The listing builds one solid part. Answer for the finished solid, in the listing's coordinates (mm). A direction names the side the tool comes from. Coordinates: 2 decimals unless noted, no trailing zeros. Order: outer loops, then holes, each group sorted by start corner. A loop starts at its lowest first (then second) coordinate and runs counter-clockwise, first axis right, second up. Notation, with made-up numbers: (-39, 44) -> (11, 44) arc R22 ccw to (11, 80) -> close; hole circle Ø4 at (68, 18.5). An arc over 180 degrees is marked (long way). Put each result on its own line as item: value. Start each with the question number.
```python
from build123d import *

# Parameters (mm, degrees)
CUT_EXTRUDE1_START = -2.681222
CUT_EXTRUDE1_DEPTH = 2.681222
CIRPATTERN3_COUNT  = 10
CUT_EXTRUDE2_REACH = 4.151
SKETCH5_R          = 2.323


with BuildPart() as part:
    # Sketch2 → Revolve2 (revolve)
    with BuildSketch(Plane(origin=(0, 0, 0), x_dir=(0, 0, -1), z_dir=(1, 0, 0))):
        Polygon((0, 0), (-7.8982, 0), (-9.91802604, 2.01982604), (-8.078303901, 3.859548179), (-6.369990486, 2.151234764), (0, 2.151234764), align=None)
    revolve(axis=Axis((0, 2.151234764, 0), (0, -1, 0)))

    # Sketch4 → Cut-Extrude1 (cut)
    with BuildSketch(Plane(origin=(-3.9491, -3.9491, 0), x_dir=(0, 0, 1), z_dir=(-0.707106781, -0.707106781, 0)).offset(CUT_EXTRUDE1_START)):
        with BuildLine():
            Line((-1.1615, 6.535539097), (1.1615, 6.535539097))
            ThreePointArc((1.1615, 6.535539097), (1.823938006, 9.981104914), (3.7168, 12.935393557))
            Line((3.7168, 12.935393557), (-3.7168, 12.935393557))
            ThreePointArc((-3.7168, 12.935393557), (-1.823938006, 9.981104914), (-1.1615, 6.535539097))
        make_face()
    cut_extrude1 = extrude(amount=CUT_EXTRUDE1_DEPTH, mode=Mode.SUBTRACT)

    # CirPattern3: Cut-Extrude1 ×10 about axis
    cirpattern3_axis = Axis((0, 0, 0), (0, 1, 0))
    for i in range(1, CIRPATTERN3_COUNT):
        add(cut_extrude1.rotate(cirpattern3_axis, i * 360 / CIRPATTERN3_COUNT), mode=Mode.SUBTRACT)

    # Sketch5 → Cut-Extrude2 (cut, up to next)
    with BuildSketch(Plane(origin=(0, 2.151234764, 0), x_dir=(1, 0, 0), z_dir=(0, 1, 0)), mode=Mode.PRIVATE) as cut_extrude2_sk1:
        Circle(SKETCH5_R)
    cut_extrude2_tool1 = extrude(cut_extrude2_sk1.sketch, amount=-CUT_EXTRUDE2_REACH, mode=Mode.PRIVATE) & part.part
    add(cut_extrude2_tool1.solids().sort_by_distance((0, 2.151235, 0))[0], mode=Mode.SUBTRACT)


solid = part.part
```
(1) For a pull along Z with two mould halves and no side action, classify faces 1 (the conical face through (-8.552, 2.953, -2.755)), 2 (the flat face through (2, 0, -2)), 3 (the cylindrical face through (8.25, 2.32, 1.21)) as released by +Z, released by -Z, zero draft, split by the parting line, or undercut.
(2) Each of these flat-tipped pins is pushed along its axis until it touches: P1, Ø6, axis at x = -5, z = 5.5, coming from the +Y side; P2, Ø1.5, axis at x = -1.5, y = 1, coming from the +Z side; P3, Ø1, axis at y = 3.5, z = -5.5, coming from the +X side; P4, Ø4, axis at x = 0, z = 0, coming from the -Y side. Where does it stop, or does it pass through?
(3) The part is cut by section C-C on y = 2.95. Count the separate pieces of the cut face and the enclosed holes in it, plus the area to 3 significant figures.
(4) The part is cut by section A-A on x = 0. Determine the outline of the cut face in (y, z).
(5) A tool of negligible diameter and unlimited length cuts with its end or side. For faces 4 (the flat face through (3, 2.151, 0)), 5 (the cylindrical face through (3.7, 2.316, -7.476)), 6 (the cylindrical face through (-3.7, 2.316, 7.476)), 7 (the cylindrical face through (5.97, 2.32, 5.83)), from which of +Z, -Z, +X, -X, +Y, -Y can it reach the whole face along a straight path? Write none if from no direction.
(6) Find the intervals of material crossed by L1, parallel to X at y = 1.8, z = 7.5; L2, parallel to X at y = 2.25, z = -4; L3, parallel to Z at x = 0, y = 0.5, in increasing order.
(7) The part is cut by section B-B on z = 0. Determine the outline of the cut face in (x, y).
Worked out:
1. face 1: released by -Z
1. face 2: zero draft
1. face 3: undercut
2. P1: y = 3.86
2. P2: z = 9.54
2. P3: x = 5.98
2. P4: through
3. separate pieces: 10
3. enclosed holes: 0
3. area: 46.8 mm2
4. outline: (0, -7.9) -> (2.02, -9.92) -> (3.86, -8.08) -> (2.15, -6.37) -> (2.15, -2.32) -> (0, -2.32) -> close; (0, 2.32) -> (2.15, 2.32) -> (2.15, 6.37) -> (3.86, 8.08) -> (2.02, 9.92) -> (0, 7.9) -> close
5. face 4: +Y
5. face 5: -Z, +Y
5. face 6: +Z, +Y
5. face 7: +X, +Y
6. L1: -6.15 to -3.68, -1.22 to 1.22, 3.68 to 6.15
6. L2: -8.82 to -7.58, -5.74 to -5.08, 5.08 to 5.74, 7.58 to 8.82
6. L3: -8.4 to -2.32, 2.32 to 8.4
7. outline: (-8.57, 0.67) -> (-7.9, 0) -> (-2.32, 0) -> (-2.32, 2.15) -> (-6.37, 2.15) -> (-6.73, 2.51) -> close; (2.32, 0) -> (7.9, 0) -> (8.57, 0.67) -> (6.73, 2.51) -> (6.37, 2.15) -> (2.32, 2.15) -> close
